Model file for the job. Use its own axes, mm. A direction names the side the tool comes from. Round coordinates to 2 decimals unless told otherwise and drop trailing zeros. Loops run counter-clockwise (first coordinate to the right, second up) from the corner with the lowest first, then second, coordinate; pieces in that order, holes last.
from build123d import *

# Parameters (mm, degrees)
SKETCH1_R           = 60
BOSS_EXTRUDE1_DEPTH = 20
SKETCH3_R           = 4
BOSS_EXTRUDE2_DEPTH = 20
SKETCH2_R           = 40
CUT_EXTRUDE1_DEPTH  = 10
SKETCH5_R           = 12
CUT_EXTRUDE2_DEPTH  = 5


with BuildPart() as part:
    # Sketch1 → Boss-Extrude1 (new body)
    with BuildSketch(Plane(origin=(0, 0, 0), x_dir=(1, 0, 0), z_dir=(0, 1, 0))):
        with Locations(Location((0, 0, 0), (0, 0, 270))):
            Circle(SKETCH1_R)
    extrude(amount=BOSS_EXTRUDE1_DEPTH)

    # Sketch3 → Boss-Extrude2 (add)
    with BuildSketch(Plane(origin=(0, 0, 0), x_dir=(1, 0, 0), z_dir=(0, 1, 0))):
        with BuildLine():
            Line((-82.857142857, 27.105237087), (-25.714285714, 54.210474174))
            ThreePointArc((-25.714285714, 54.210474174), (60, 0), (-25.714285714, -54.210474174))
            Line((-25.714285714, -54.210474174), (-82.857142857, -27.105237087))
            ThreePointArc((-82.857142857, -27.105237087), (-100, 0), (-82.857142857, 27.105237087))
        make_face()
        with Locations(Location((-70, 0, 0), (0, 0, 270))):
            Circle(SKETCH3_R, mode=Mode.SUBTRACT)
    extrude(amount=BOSS_EXTRUDE2_DEPTH)

    # Sketch2 → Cut-Extrude1 (cut)
    with BuildSketch(Plane(origin=(0, 20, 0), x_dir=(1, 0, 0), z_dir=(0, 1, 0))):
        with Locations(Location((0, 0, 0), (0, 0, 270))):
            Circle(SKETCH2_R)
    extrude(amount=-CUT_EXTRUDE1_DEPTH, mode=Mode.SUBTRACT)

    # Sketch5 → Cut-Extrude2 (cut)
    with BuildSketch(Plane.XZ):
        with Locations(Location((-70, 0, 0), (0, 0, 270))):
            Circle(SKETCH5_R)
    extrude(amount=-CUT_EXTRUDE2_DEPTH, mode=Mode.SUBTRACT)


solid = part.part
Q1. Pull direction Z, two halves, no side cores. Call faces 4 (the face through (59.976, 9.86, 1.691)), 5 (the face through (-39.05, 15.07, -8.67)), 6 (the face through (-19, 0, -1)), 7 (the face through (-81.715, 2.465, 2.601)): pulls with the +Z half, pulls with the -Z half, needs draft (parallel to the pull), parting line crosses it, or undercut.
Q2. Slice it at D-D on y = 2. Give the cut face in (x, z).
Q3. Flat gauge pins, fed straight in: P1, Ø4, axis at y = 13, z = 47.5, coming from the +X side; P2, Ø7, axis at x = -65.5, z = -4.5, coming from the -Y side; P3, Ø1, axis at y = 5.5, z = 24, coming from the -X side. Where does each tip first touch, or does it go through?
Q4. Slice it at A-A on z = 0. Give the cut face in (x, y).
Q5. Slice it at B-B on x = 0. Give the cut face in (y, z), plus the area to 3 significant figures.
Q6. Slice it at C-C on y = 17. Give the cut face in (x, z), plus the area to 3 significant figures.
Q7. Tool access for faces 1 (the face through (-67, 5, 3)), 2 (the face through (1, 10, -1)), 3 (the face through (-37, 20, 26)): list every direction of +Z, -Z, +X, -X, +Y, -Y with a clear straight run to the whole face (end or side of a thin tool).
Q8. Probe line 1 (X direction, y = 17.75, z = 0); line 2 (X direction, y = 1.6, z = 0); line 3 (Y direction, x = 23.5, z = 31). List the from-to ranges inside material, lowest first.
Reply:
1. face 4: parting line crosses it
1. face 5: undercut
1. face 6: needs draft
1. face 7: undercut
2. outline: (-82.86, -27.11) - (-25.71, -54.21) arc R60 ccw (long way) to (-25.71, 54.21) - (-82.86, 27.11) arc R30 ccw to start; hole circle Ø24 at (-70, 0)
3. P1: stops at x = 39.11
3. P2: stops at y = 5
3. P3: stops at x = -88.65
4. outline: (-100, 0) - (-82, 0) - (-82, 5) - (-74, 5) - (-74, 20) - (-100, 20) - close; (-66, 5) - (-58, 5) - (-58, 0) - (60, 0) - (60, 20) - (40, 20) - (40, 10) - (-40, 10) - (-40, 20) - (-66, 20) - close
5. outline: (0, -60) - (20, -60) - (20, -40) - (10, -40) - (10, 40) - (20, 40) - (20, 60) - (0, 60) - close
5. area: 1,600 mm2
6. outline: (-82.86, -27.11) - (-25.71, -54.21) arc R60 ccw (long way) to (-25.71, 54.21) - (-82.86, 27.11) arc R30 ccw to start; hole circle Ø8 at (-70, 0); hole circle Ø80 at (0, 0)
6. area: 8,880 mm2
7. face 1: -Y
7. face 2: +Y
7. face 3: +Z, -Z, +X, -X, +Y
8. line 1: x = -100 to -74, -66 to -40, 40 to 60
8. line 2: x = -100 to -82, -58 to 60
8. line 3: y = 0 to 10
